Source: three-view drawing plus pictorial views. Frame: mm from the lowest corner of the part. A direction names the side the tool comes from. Coordinates: 2 decimals unless noted, no trailing zeros. Loops run counter-clockwise (first coordinate to the right, second up) from the corner with the lowest first, then second, coordinate; pieces in that order, holes last.
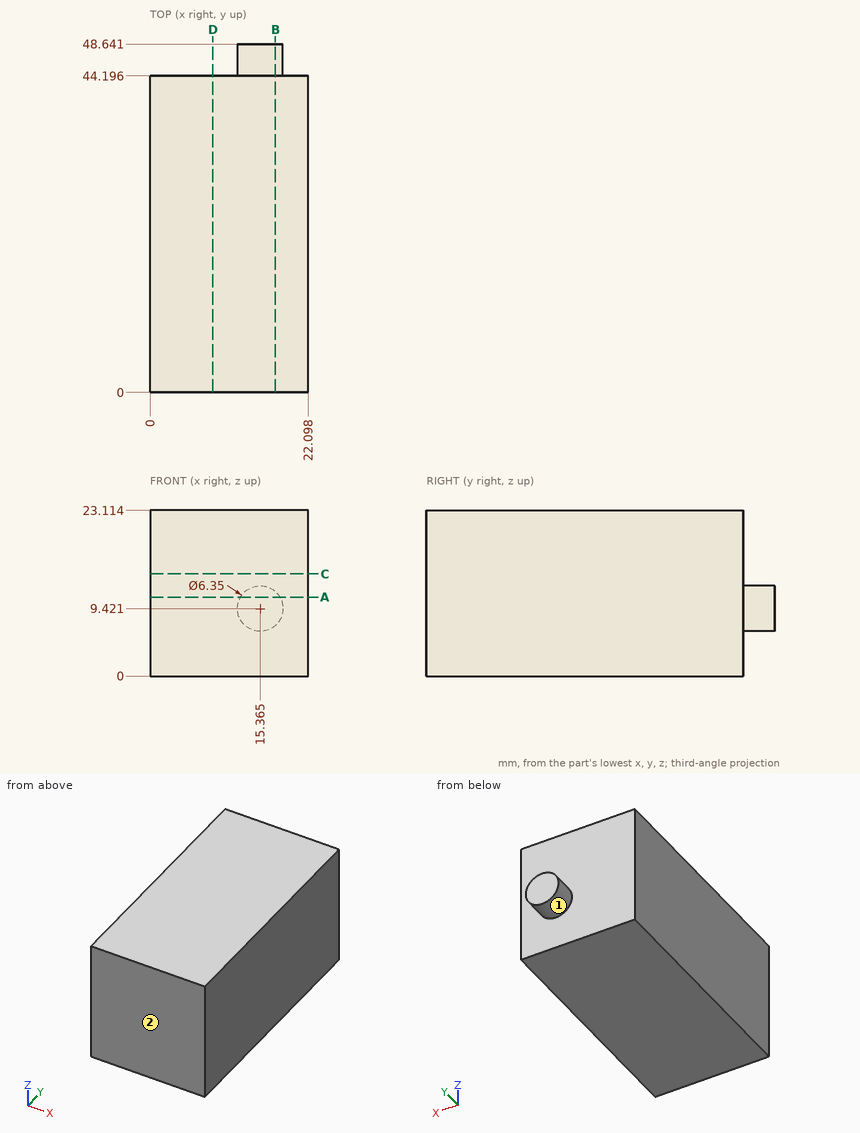
Q1. Section query B-B on x = 17.5. Return the cut outline in (y, z).
Q2. Reachability of the marked faces 1 and 2 from +Z, -Z, +X, -X, +Y, -Y: full face, straight path, thin tool, end or side. Return the list, or none.
Q3. First-contact query: pin 1 Ø1 at (x, z) = (4, 4) entering from +Y. Flat tip, straight axial feed; report the tip coordinate or a pass-through.
Q4. Material intervals for line 1 along Y through (x, z) = (14.25, 20.25), sorted ascending.
Q5. Section query A-A on z = 11. Return the cut outline in (x, y), then the cut area to 3 significant figures.
Q6. Section query C-C on z = 14.25. Return the cut outline in (x, y).
Q7. Section query D-D on x = 8.75. Return the cut outline in (y, z), then the cut area to 3 significant figures.
Resolved:
1. outline: (0, 0) - (44.2, 0) - (44.2, 7.07) - (48.64, 7.07) - (48.64, 11.77) - (44.2, 11.77) - (44.2, 23.11) - (0, 23.11) - close
2. face 1: +Y
2. face 2: +Z, -Z, +X, -X, -Y
3. pin 1: stops at y = 44.2
4. line 1: y = 0 to 44.2
5. outline: (0, 0) - (22.1, 0) - (22.1, 44.2) - (18.12, 44.2) - (18.12, 48.64) - (12.61, 48.64) - (12.61, 44.2) - (0, 44.2) - close
5. area: 1,000 mm2
6. outline: (0, 0) - (22.1, 0) - (22.1, 44.2) - (0, 44.2) - close
7. outline: (0, 0) - (44.2, 0) - (44.2, 23.11) - (0, 23.11) - close
7. area: 1,020 mm2
